Geometry: see drawing. Coordinates: mm, zero at the bounding-box minimum. Round coordinates to 2 decimals unless told otherwise and drop trailing zeros. Loops run counter-clockwise (first coordinate to the right, second up) from the corner with the lowest first, then second, coordinate; pieces in that order, holes last.
(1) First-contact query: pin 1 Ø6 at (y, z) = (7.94, 19.05) entering from +X. Flat tip, straight axial feed; report the tip coordinate or a pass-through.
(2) Cut plane B-B, the plane z = 16.5. Output: boundary loops of the cut face in (x, y) (1 decimal).
(3) Line query: line 1 (Y direction, x = 1.2, z = 19.05) (1 decimal); line 2 (Z direction, x = 0.9, y = 9) (1 decimal); line 3 (Z direction, x = 0.3, y = 9.75) (1 decimal). Output: solid intervals per line, ascending.
(4) Cut plane D-D, the plane y = 3.25. Output: boundary loops of the cut face in (x, z) (1 decimal).
(5) Cut plane A-A, the plane y = 6.25. Output: boundary loops of the cut face in (x, z).
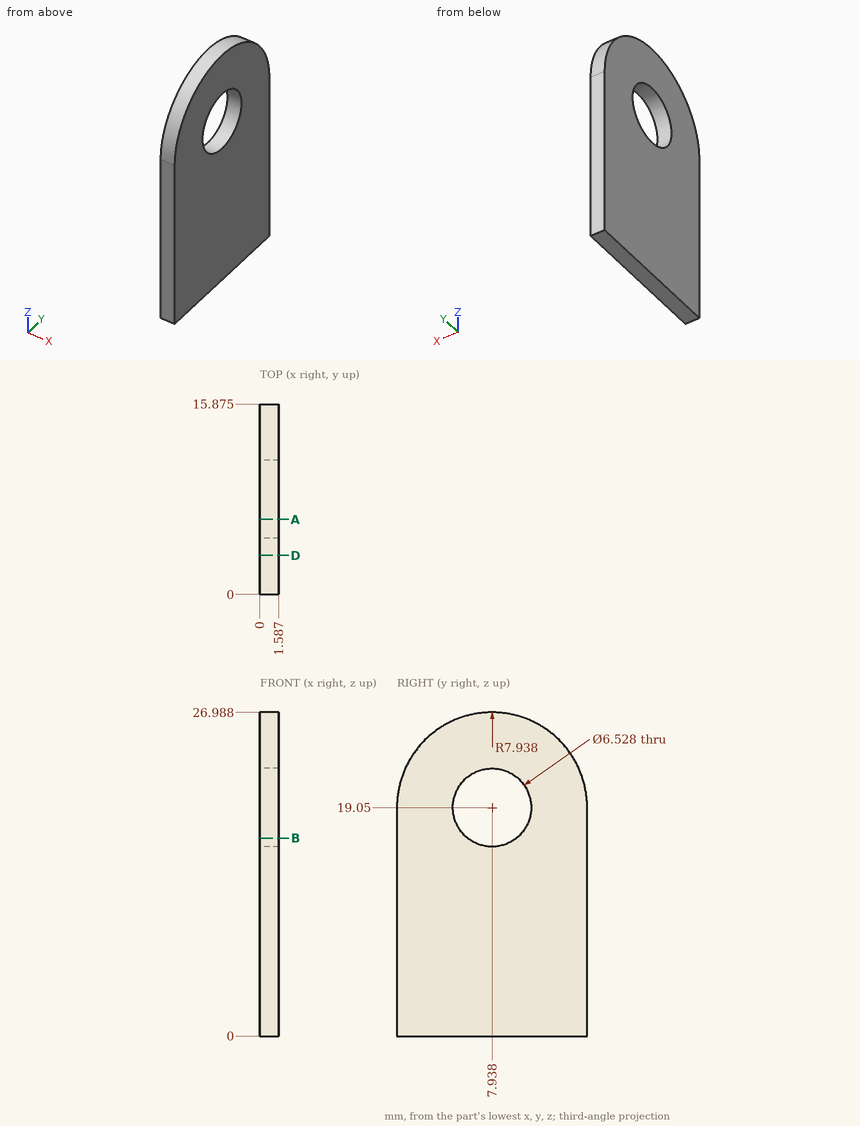
Reported:
1. pin 1: passes through
2. outline: (0, 0) - (1.6, 0) - (1.6, 5.9) - (0, 5.9) - close; (0, 10) - (1.6, 10) - (1.6, 15.9) - (0, 15.9) - close
3. line 1: y = 0 to 4.7, 11.2 to 15.9
3. line 2: z = 0 to 16, 22.1 to 26.9
3. line 3: z = 0 to 16.3, 21.8 to 26.8
4. outline: (0, 0) - (1.6, 0) - (1.6, 25.5) - (0, 25.5) - close
5. outline: (0, 0) - (1.59, 0) - (1.59, 16.26) - (0, 16.26) - close; (0, 21.84) - (1.59, 21.84) - (1.59, 26.81) - (0, 26.81) - close
